Work out the finished part from the listing and answer in its coordinate system (mm). Face numbers are marked on the shaded views. Round coordinates to 2 decimals unless told otherwise and drop trailing zeros. Write each loop counter-clockwise with the first axis right and the second up, starting at its lowest first coordinate (ties: lowest second). Pieces come first, ordered by that corner, then holes. Notation, with made-up numbers: (73.25, 63.25) -> (130.25, 63.25) arc R32 ccw to (130.25, 95.25) -> close; hole circle Ø2 at (12, 29.5). An arc over 180 degrees is marked (long way). One line per item, written item: value.
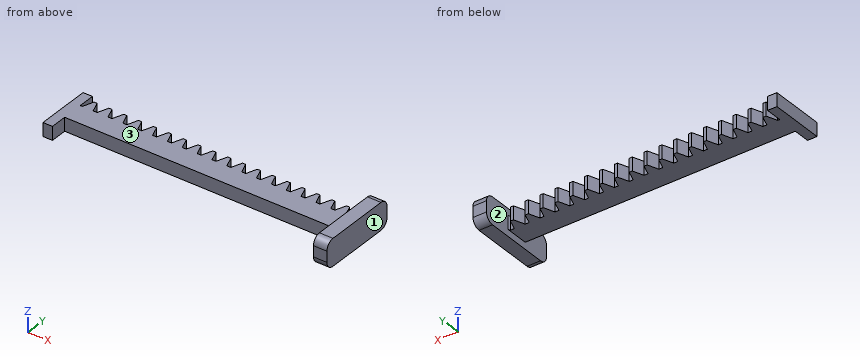
```python
from build123d import *

# Parameters (mm, degrees)
BLANKSKE_W         = 100
BLANKSKE_H         = 11.75
BLANK_DEPTH        = 5
TOOTHCUTSIM_DEPTH  = 101.812015653
TEETHCUTS_COUNT    = 19
TEETHCUTS_PITCH    = 5.497787138
ESQUISSE1_W        = 3.5
ESQUISSE1_H        = 20
BOSS_EXTRU_1_DEPTH = 5
BOSS_EXTRU_2_DEPTH = 5


with BuildPart() as part:
    # BlankSke → Blank (new body)
    with BuildSketch(Plane.XY):
        with Locations((50, 5.875)):
            Rectangle(BLANKSKE_W, BLANKSKE_H)
    extrude(amount=-BLANK_DEPTH)

    # TooCutSkeSim → ToothCutSim (cut, through all)
    with BuildSketch(Plane.XY):
        Polygon((0.737261897, 7.8125), (-0.737261897, 7.8125), (-2.179639538, 11.7754), (2.179639538, 11.7754), align=None)
    toothcutsim = extrude(amount=-TOOTHCUTSIM_DEPTH, mode=Mode.SUBTRACT)

    # TeethCuts: ToothCutSim ×19
    with Locations(*[(i * TEETHCUTS_PITCH, 0, 0) for i in range(1, TEETHCUTS_COUNT)]):
        add(toothcutsim, mode=Mode.SUBTRACT)

    # Esquisse1 → Boss.-Extru.1 (add, through all)
    with BuildSketch(Plane(origin=(0, 0, -5), x_dir=(-1, 0, 0), z_dir=(0, 0, -1))):
        with Locations((1.75, 3.90625)):
            Rectangle(ESQUISSE1_W, ESQUISSE1_H)
    extrude(amount=-BOSS_EXTRU_1_DEPTH)

    # Esquisse4 → Boss.-Extru.2 (add)
    with BuildSketch(Plane(origin=(100, 0, 0), x_dir=(0, 0, -1), z_dir=(1, 0, 0))):
        with BuildLine():
            Line((0.5, -10.67809839), (4.5, -10.67809839))
            ThreePointArc((4.5, -10.67809839), (6.621320344, -9.799418733), (7.5, -7.67809839))
            Line((7.5, -7.67809839), (7.5, 16.32190161))
            ThreePointArc((7.5, 16.32190161), (6.621320344, 18.443221954), (4.5, 19.32190161))
            Line((4.5, 19.32190161), (0.5, 19.32190161))
            ThreePointArc((0.5, 19.32190161), (-1.621320344, 18.443221954), (-2.5, 16.32190161))
            Line((-2.5, 16.32190161), (-2.5, -7.67809839))
            ThreePointArc((-2.5, -7.67809839), (-1.621320344, -9.799418733), (0.5, -10.67809839))
        make_face()
    extrude(amount=BOSS_EXTRU_2_DEPTH)


solid = part.part
```
(1) Find section B-B on y = 4. Give the vertices of the cut face in (x, z), plus the area to 4 significant figures.
Reported:
outline: (-3.5, -5) -> (100, -5) -> (100, -7.5) -> (105, -7.5) -> (105, 2.5) -> (100, 2.5) -> (100, 0) -> (-3.5, 0) -> close
area: 567.5 mm2
(2) Consider probe 1 along X at (y, z) = (13.5, -3.25); probe 2 along Z at (x, y) = (79, 0.75); probe 3 along X at (y, z) = (13, 2). Determine where each line is inside the solid, lowest interval first.
Reported:
probe 1: x = -3.5 to 0, 100 to 105
probe 2: z = -5 to 0
probe 3: x = 100 to 105
(3) Find section A-A on y = -1. Give the vertices of the cut face in (x, z).
Reported:
outline: (-3.5, -5) -> (0, -5) -> (0, 0) -> (-3.5, 0) -> close; (100, -7.5) -> (105, -7.5) -> (105, 2.5) -> (100, 2.5) -> close
(4) Flat-ended cylindrical pins translate along their axes: pin 1 Ø0.9 at (x, z) = (41, -1.5) entering from +Y; pin 2 Ø1.5 at (x, z) = (70.5, -5) entering from -Y; pin 3 Ø1.2 at (x, z) = (71.5, -3) entering from +Y. Find the tip coordinate at first contact, or state that the pin passes through.
Reported:
pin 1: stops at y = 11.75
pin 2: stops at y = 0
pin 3: stops at y = 7.81
(5) For a pull along X with two mould halves and no side action, classify the marked faces 1, 2 and 3 as pulls with the +X half, pulls with the -X half, needs draft (parallel to the pull), parting line crosses it, or undercut.
Reported:
face 1: pulls with the +X half
face 2: undercut
face 3: needs draft
